Input: part model. Units: mm. Frame: model coordinates. A direction names the side the tool comes from. Round coordinates to 2 decimals unless told otherwise and drop trailing zeros. Loops run counter-clockwise (first coordinate to the right, second up) from the corner with the lowest first, then second, coordinate; pieces in that order, holes last. Notation, with made-up numbers: (74.5, 13.25) - (85.5, 13.25) arc R22 cw to (85.5, 32.25) - close; hole circle Ø6 at (85, 81.5). An arc over 180 degrees is marked (long way). Write each question's results on one line, items separated by ' | '.
Autodesk Inventor part; units mm, degrees
ref_plane "Начальная плоскость" through (0, 0, 0) normal (0, 0, 1) x (1, 0, 0)
ref_plane "Конечная плоскость" through (0, 0, 38) normal (0, 0, 1) x (1, 0, 0)
ref_plane "РабПлоскость4" through (-10, 0, 38) normal (0.7071, 0, 0.7071) x (0.7071, 0, -0.7071)
ref_plane "Начальная плоскость" through (0, 0, 0) normal (0, 0, 1) x (1, 0, 0)
ref_plane "Конечная плоскость" through (0, 0, 38) normal (0, 0, 1) x (1, 0, 0)
sketch "Эскиз" plane through (0, 0, 0) normal (0, 0, 1) x (1, 0, 0)
  line L0 (-14.4349, 0) -> (14.4349, 0)
  line L1 (0, -14) -> (0, 14)
  line L2 (0, 0) -> (7.5, 7.5) construction
  circle A0 centre (7.5, 7.5) radius 1.65 construction
  line L3 (5.85, 9.15) -> (9.15, 9.15)
  line L4 (9.15, 9.15) -> (9.15, 5.85)
  line L5 (9.15, 5.85) -> (5.85, 5.85)
  line L6 (5.85, 5.85) -> (5.85, 9.15)
  line L7 (3.235, 8.1636) -> (4.72, 9.9636)
  line L8 (4.7971, 10) -> (8.5, 10)
  line L9 (3.3121, 8) -> (4.95, 8)
  line L10 (4.95, 8) -> (4.95, 5.7985)
  line L11 (4.95, 5.7985) -> (2.6515, 3.5)
  line L12 (0, 3.5) -> (2.6515, 3.5)
  circle A1 centre (0, 0) radius 2.5
  line L13 (8.1636, 3.235) -> (9.9636, 4.72)
  line L14 (10, 4.7971) -> (10, 8.5)
  line L15 (8, 3.3121) -> (8, 4.95)
  line L16 (8, 4.95) -> (5.7985, 4.95)
  line L17 (5.7985, 4.95) -> (3.5, 2.6515)
  line L18 (3.5, 0) -> (3.5, 2.6515)
  arc A2 (10, 8.5) -> (8.5, 10) centre (8.5, 8.5) ccw
  line L19 (0, 0) -> (-7.5, 7.5) construction
  circle A3 centre (-7.5, 7.5) radius 1.65 construction
  line L20 (-5.85, 9.15) -> (-9.15, 9.15)
  line L21 (-9.15, 9.15) -> (-9.15, 5.85)
  line L22 (-9.15, 5.85) -> (-5.85, 5.85)
  line L23 (-5.85, 5.85) -> (-5.85, 9.15)
  line L24 (-3.235, 8.1636) -> (-4.72, 9.9636)
  line L25 (-4.7971, 10) -> (-8.5, 10)
  line L26 (-3.3121, 8) -> (-4.95, 8)
  line L27 (-4.95, 8) -> (-4.95, 5.7985)
  line L28 (-4.95, 5.7985) -> (-2.6515, 3.5)
  line L29 (0, 3.5) -> (-2.6515, 3.5)
  line L30 (-3.5, 0) -> (-3.5, 2.6515)
  line L31 (-5.7985, 4.95) -> (-3.5, 2.6515)
  line L32 (-8, 4.95) -> (-5.7985, 4.95)
  line L33 (-8, 3.3121) -> (-8, 4.95)
  line L34 (-8.1636, 3.235) -> (-9.9636, 4.72)
  line L35 (-10, 4.7971) -> (-10, 8.5)
  arc A4 (-8.5, 10) -> (-10, 8.5) centre (-8.5, 8.5) ccw
  line L36 (0, 14) -> (0, -14)
  line L37 (0, 0) -> (7.5, -7.5) construction
  circle A5 centre (7.5, -7.5) radius 1.65 construction
  line L38 (5.85, -9.15) -> (9.15, -9.15)
  line L39 (9.15, -9.15) -> (9.15, -5.85)
  line L40 (9.15, -5.85) -> (5.85, -5.85)
  line L41 (5.85, -5.85) -> (5.85, -9.15)
  line L42 (3.235, -8.1636) -> (4.72, -9.9636)
  line L43 (4.7971, -10) -> (8.5, -10)
  line L44 (3.3121, -8) -> (4.95, -8)
  line L45 (4.95, -8) -> (4.95, -5.7985)
  line L46 (4.95, -5.7985) -> (2.6515, -3.5)
  line L47 (0, -3.5) -> (2.6515, -3.5)
  line L48 (3.5, 0) -> (3.5, -2.6515)
  line L49 (5.7985, -4.95) -> (3.5, -2.6515)
  line L50 (8, -4.95) -> (5.7985, -4.95)
  line L51 (8, -3.3121) -> (8, -4.95)
  line L52 (8.1636, -3.235) -> (9.9636, -4.72)
  line L53 (10, -4.7971) -> (10, -8.5)
  arc A6 (8.5, -10) -> (10, -8.5) centre (8.5, -8.5) ccw
  line L54 (0, 0) -> (-7.5, -7.5) construction
  line L55 (-4.95, -8) -> (-4.95, -5.7985)
  line L56 (-3.3121, -8) -> (-4.95, -8)
  line L57 (-5.7985, -4.95) -> (-3.5, -2.6515)
  line L58 (-4.95, -5.7985) -> (-2.6515, -3.5)
  line L59 (-3.5, 0) -> (-3.5, -2.6515)
  line L60 (0, -3.5) -> (-2.6515, -3.5)
  circle A7 centre (-7.5, -7.5) radius 1.65 construction
  line L61 (-5.85, -5.85) -> (-5.85, -9.15)
  line L62 (-5.85, -9.15) -> (-9.15, -9.15)
  line L63 (-9.15, -9.15) -> (-9.15, -5.85)
  line L64 (-9.15, -5.85) -> (-5.85, -5.85)
  line L65 (-3.235, -8.1636) -> (-4.72, -9.9636)
  line L66 (-8, -4.95) -> (-5.7985, -4.95)
  line L67 (-8, -3.3121) -> (-8, -4.95)
  line L68 (-8.1636, -3.235) -> (-9.9636, -4.72)
  line L69 (-4.7971, -10) -> (-8.5, -10)
  line L70 (-10, -4.7971) -> (-10, -8.5)
  arc A8 (-10, -8.5) -> (-8.5, -10) centre (-8.5, -8.5) ccw
  arc A9 (3.235, 8.1636) -> (3.3121, 8) centre (3.3121, 8.1) ccw
  arc A10 (4.7971, 10) -> (4.72, 9.9636) centre (4.7971, 9.9) ccw
  arc A11 (8, 3.3121) -> (8.1636, 3.235) centre (8.1, 3.3121) ccw
  arc A12 (9.9636, 4.72) -> (10, 4.7971) centre (9.9, 4.7971) ccw
  arc A13 (-3.3121, 8) -> (-3.235, 8.1636) centre (-3.3121, 8.1) ccw
  arc A14 (-4.72, 9.9636) -> (-4.7971, 10) centre (-4.7971, 9.9) ccw
  arc A15 (-8.1636, 3.235) -> (-8, 3.3121) centre (-8.1, 3.3121) ccw
  arc A16 (-10, 4.7971) -> (-9.9636, 4.72) centre (-9.9, 4.7971) ccw
  arc A17 (-8, -3.3121) -> (-8.1636, -3.235) centre (-8.1, -3.3121) ccw
  arc A18 (-9.9636, -4.72) -> (-10, -4.7971) centre (-9.9, -4.7971) ccw
  arc A19 (-3.235, -8.1636) -> (-3.3121, -8) centre (-3.3121, -8.1) ccw
  arc A20 (-4.7971, -10) -> (-4.72, -9.9636) centre (-4.7971, -9.9) ccw
  arc A21 (4.72, -9.9636) -> (4.7971, -10) centre (4.7971, -9.9) ccw
  arc A22 (3.3121, -8) -> (3.235, -8.1636) centre (3.3121, -8.1) ccw
  arc A23 (8.1636, -3.235) -> (8, -3.3121) centre (8.1, -3.3121) ccw
  arc A24 (10, -4.7971) -> (9.9636, -4.72) centre (9.9, -4.7971) ccw
  point P0 (3.1, 8)
  point P1 (4.75, 10)
  point P2 (7.5, 9.15)
  point P3 (8, 3.1)
  point P4 (10, 4.75)
  point P5 (7.5, 5.85)
  point P6 (9.15, 7.5)
  point P7 (-3.1, 8)
  point P8 (-4.75, 10)
  point P9 (-7.5, 9.15)
  point P10 (-8, 3.1)
  point P11 (-10, 4.75)
  point P12 (-7.5, 5.85)
  point P13 (-9.15, 7.5)
  point P14 (3.1, -8)
  point P15 (4.75, -10)
  point P16 (7.5, -9.15)
  point P17 (8, -3.1)
  point P18 (10, -4.75)
  point P19 (7.5, -5.85)
  point P20 (9.15, -7.5)
  point P21 (-3.1, -8)
  point P22 (-7.5, -5.85)
  point P23 (-7.5, -9.15)
  point P24 (-9.15, -7.5)
  point P25 (-4.75, -10)
  point P26 (-8, -3.1)
  point P27 (-10, -4.75)
  dimension "d0" = 45
  dimension "d1" = 3.3
  dimension "d2" = 1.5
  dimension "d3" = 1.2
  dimension "d4" = 5
  dimension "d5" = 6.5
  dimension "d6" = 15
  dimension "d7" = 20
  dimension "d8" = 9.9
  dimension "d9" = 9.5
  dimension "d10" = 6.2
  dimension "d11" = 2
  dimension "d18" = 0.1
  dimension "d19" = 0.1
extrude "Тело" add sketch "Эскиз" along normal up to surface (38 mm away) from surface at 0 contours A1 L1 L12 L11 L10 L9 A9 L7 A10 L8 A2 L14 A12 L13 A11 L15 L16 L17 L18 L0 | L0 L48 L49 L50 L51 A23 L52 A24 L53 A6 L43 A21 L42 A22 L44 L45 L46 L47 L1 A1 | A1 L0 L30 L31 L32 L33 A15 L34 A16 L35 A4 L25 A14 L24 A13 L26 L27 L28 L29 L1 | L1 L60 L58 L55 L56 A19 L65 A20 L69 A8 L70 A18 L68 A17 L67 L66 L57 L59 L0 A1
sketch "Эскиз2" plane through (0, 0, 0) normal (0, 0, 1) x (1, 0, 0)
  line L0 (0, 0) -> (10, 0)
ref_plane "РабПлоскость3" through (0, 0, 0) normal (0, -1, 0) x (1, 0, 0)
sketch "Эскиз3" plane through (0, 0, 0) normal (0, -1, 0) x (1, 0, 0)
  line L0 (-2, 0) -> (12, 0)
  line L1 (-2, 38) -> (12, 38)
  dimension "d25" = 38
ref_plane "РабПлоскость4" through (-10, 0, 38) normal (0.7071, 0, 0.7071) x (0.7071, 0, -0.7071)
split "Разделение1" plane through (-10, 0, 38) removes the side toward (0.7071, 0, 0.7071)
equation "\"Длина\" = 28"
equation "\"G_OFFSET_START\" = 0"
equation "\"d21\" = Длина + G_OFFSET_END"
equation "\"G_L\" = d25"
properties part number "короткая палка"
1. Section query A-A, the plane x = 0. Output: boundary loops of the cut face in (y, z).
Answer:
outline: (-3.5, 0) - (-2.5, 0) - (-2.5, 28) - (-3.5, 28) - close; (2.5, 0) - (3.5, 0) - (3.5, 28) - (2.5, 28) - close
2. Section query B-B, the plane y = -7.25. Output: boundary loops of the cut face in (x, z), plus the area to 3 significant figures.
Answer:
outline: (-10, 0) - (-9.15, 0) - (-9.15, 37.15) - (-10, 38) - close; (-5.85, 0) - (-4.95, 0) - (-4.95, 32.95) - (-5.85, 33.85) - close; (4.95, 0) - (5.85, 0) - (5.85, 22.15) - (4.95, 23.05) - close; (9.15, 0) - (10, 0) - (10, 18) - (9.15, 18.85) - close | area: 98.0 mm^2
3. Mould query, pull axis Y, two halves, no side actions, for faces 1 (the flat face through (-7, 10, 18)), 2 (the flat face through (4.95, -7, 11)), 3 (the flat face through (10, 7, 9)). Classes: pulls with the +Y half, pulls with the -Y half, needs draft (parallel to the pull), parting line crosses it, or undercut.
Answer:
face 1: pulls with the +Y half | face 2: undercut | face 3: needs draft
4. Set-up query: faces 4 (the flat face through (4.67, -3.82, 12.08)), 5 (the flat face through (-3.967, 9.051, 16.131)), 6 (the flat face through (9.051, 3.967, 9.779)). Return all of +Z, -Z, +X, -X, +Y, -Y with unobstructed straight access to the full face (end or side cutting, diameter ignored); none if empty.
Answer:
face 4: +Z, -Z | face 5: +Z, -Z, +Y | face 6: +Z, -Z, +X
5. Section query C-C, the plane x = 7.5. Output: boundary loops of the cut face in (y, z), plus the area to 4 significant figures.
Answer:
outline: (-10, 0) - (-9.15, 0) - (-9.15, 20.5) - (-10, 20.5) - close; (-5.85, 0) - (-4.95, 0) - (-4.95, 20.5) - (-5.85, 20.5) - close; (4.95, 0) - (5.85, 0) - (5.85, 20.5) - (4.95, 20.5) - close; (9.15, 0) - (10, 0) - (10, 20.5) - (9.15, 20.5) - close | area: 71.75 mm^2
6. Contact query for flat-ended pins moving along their axis: pin 1 (5 mm diameter, centred on y = -3.5, z = 25, fed in from +X); pin 2 (0.5 mm diameter, centred on y = -4, z = 10, fed in from -X); pin 3 (1 mm diameter, centred on y = 7, z = 31, fed in from +X). Output: stop coordinate, or through.
Answer:
pin 1: x = 5.31 | pin 2: x = -9.39 | pin 3: x = -4.95
7. Line query: line 1 (X direction, y = -6.25, z = 4.5); line 2 (Y direction, x = 0, z = 11). Output: solid intervals per line, ascending. Write a range as [from, to].
Answer:
line 1: [-10, -9.15], [-5.85, -4.95], [4.95, 5.85], [9.15, 10] | line 2: [-3.5, -2.5], [2.5, 3.5]
8. Section query D-D, the plane y = 0. Output: boundary loops of the cut face in (x, z).
Answer:
outline: (-3.5, 0) - (-2.5, 0) - (-2.5, 30.5) - (-3.5, 31.5) - close; (2.5, 0) - (3.5, 0) - (3.5, 24.5) - (2.5, 25.5) - close
